```python
from build123d import *

# Parameters (mm, degrees)
SKETCH4_W            = 28.705590634
SKETCH4_H            = 208.526976526
BOSS_EXTRUDE5_DEPTH  = 20
SKETCH5_W            = 28.705590634
SKETCH5_H            = 20.449519005
SKETCH5_W_2          = 31.445291082
SKETCH5_H_2          = 18.706651284
BOSS_EXTRUDE6_DEPTH  = 40
SKETCH6_W            = 31.445291082
SKETCH6_H            = 208.079798694
BOSS_EXTRUDE7_DEPTH  = 40
SKETCH7_W            = 18.3
SKETCH7_H            = 20
CUT_EXTRUDE1_DEPTH   = 28.705590634
SKETCH8_W            = 208.079798694
SKETCH8_H            = 10.562870441
SKETCH8_H_2          = 11.993481809
BOSS_EXTRUDE8_DEPTH  = 15
SKETCH11_W           = 20
SKETCH11_H           = 32
CUT_EXTRUDE2_DEPTH   = 39
SKETCH12_W           = 21.023017078
SKETCH12_H           = 19.656473247
SKETCH12_W_2         = 18.706651284
SKETCH12_H_2         = 20
BOSS_EXTRUDE10_DEPTH = 68
SKETCH13_W           = 19.268882627
SKETCH13_H           = 20
SKETCH13_W_2         = 20.449519005
BOSS_EXTRUDE11_DEPTH = 64


with BuildPart() as part:
    # Sketch4 → Boss-Extrude5 (new body)
    with BuildSketch(Plane(origin=(0, -18, 0), x_dir=(1, 0, 0), z_dir=(0, 1, 0))):
        with Locations((-364.278541189, -59.921815566)):
            Rectangle(SKETCH4_W, SKETCH4_H)
    extrude(amount=BOSS_EXTRUDE5_DEPTH)

    # Sketch5 → Boss-Extrude6 (add)
    with BuildSketch(Plane.XZ.offset(18)):
        with Locations((-364.278541189, 153.960544327)):
            Rectangle(SKETCH5_W, SKETCH5_H)
        with Locations((-365.648391413, -34.988347055)):
            Rectangle(SKETCH5_W_2, SKETCH5_H_2)
    extrude(amount=BOSS_EXTRUDE6_DEPTH)

    # Sketch6 → Boss-Extrude7 (add)
    with BuildSketch(Plane.XZ.offset(58)):
        with Locations((-365.648391413, 60.145404482)):
            Rectangle(SKETCH6_W, SKETCH6_H)
    extrude(amount=BOSS_EXTRUDE7_DEPTH)

    # Sketch7 → Cut-Extrude1 (cut)
    with BuildSketch(Plane.ZY.offset(378.631336506)):
        with Locations((61.073274434, -8)):
            Rectangle(SKETCH7_W, SKETCH7_H)
    extrude(amount=-CUT_EXTRUDE1_DEPTH, mode=Mode.SUBTRACT)

    # Sketch8 → Boss-Extrude8 (add)
    with BuildSketch(Plane.ZY.offset(378.631336506)):
        with Locations((60.145404482, -63.281435221)):
            Rectangle(SKETCH8_W, SKETCH8_H)
        with Locations((60.145404482, -92.003259095)):
            Rectangle(SKETCH8_W, SKETCH8_H_2)
    extrude(amount=BOSS_EXTRUDE8_DEPTH)

    # Sketch11 → Cut-Extrude2 (cut)
    with BuildSketch(Plane.ZY.offset(393.631336506)):
        with Locations((145.629013926, -78.238745267)):
            Rectangle(SKETCH11_W, SKETCH11_H)
        with Locations((-23.889291997, -78.292410405)):
            Rectangle(SKETCH11_W, SKETCH11_H)
    extrude(amount=-CUT_EXTRUDE2_DEPTH, mode=Mode.SUBTRACT)

    # Sketch12 → Boss-Extrude10 (add)
    with BuildSketch(Plane.ZY.offset(378.631336506)):
        with Locations((153.67379529, -7.828236624)):
            Rectangle(SKETCH12_W, SKETCH12_H)
        with Locations((-34.988347055, -8)):
            Rectangle(SKETCH12_W_2, SKETCH12_H_2)
    extrude(amount=BOSS_EXTRUDE10_DEPTH)

    # Sketch13 → Boss-Extrude11 (add)
    with BuildSketch(Plane(origin=(-349.925745872, 0, 0), x_dir=(0, 0, -1), z_dir=(1, 0, 0))):
        with Locations((34.707231384, -8)):
            Rectangle(SKETCH13_W, SKETCH13_H)
        with Locations((-153.960544327, -8)):
            Rectangle(SKETCH13_W_2, SKETCH13_H)
    extrude(amount=BOSS_EXTRUDE11_DEPTH)


solid = part.part
```
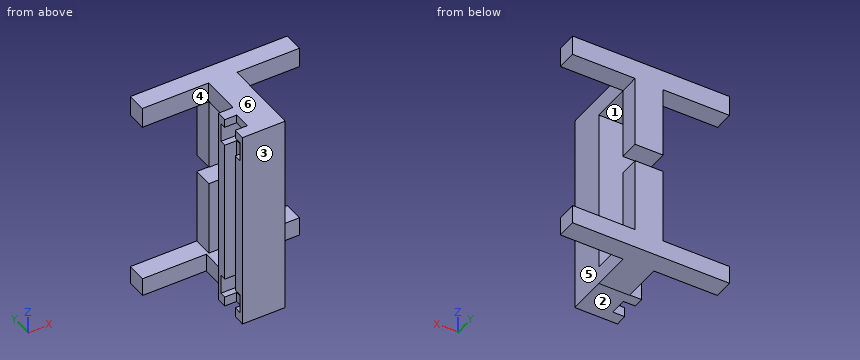
Design review of the part built by this model. Coordinates are the model's own, in mm. Face numbers are marked on the shaded views. A direction names the side the tool comes from. Round coordinates to 2 decimals unless told otherwise and drop trailing zeros. Write each loop counter-clockwise with the first axis right and the second up, starting at its lowest first coordinate (ties: lowest second). Pieces come first, ordered by that corner, then holes.
Item 1: We need section C-C on z = 22. Write out the cut boundary in (x, y).
Item 2: Clearance check with flat-ended pins moving along their axes: pin 1 Ø3 at (y, z) = (-83.5, 117.5) entering from -X; pin 2 Ø16 at (y, z) = (-3.5, 30.5) entering from +X; pin 3 Ø16 at (x, y) = (-370, -71.5) entering from -Z. State where each tip first meets the part, or that it passes through.
Item 3: We need section B-B on y = -24.5. Write out the cut boundary in (x, z), and give its area (3 significant figures).
Item 4: For the marked faces 4, 5 and 6, list the 3-axis set-ups (+Z, -Z, +X, -X, +Y, -Y) from which the entire face can be reached by the end or side of a thin tool; tool diameter is ignored.
Item 5: We need section A-A on x = -337. Write out the cut boundary in (y, z).
Item 6: The part is to be moulded in two halves that separate along Z. For the marked faces 1, 2 and 3, say which applies: +Z half, -Z half, draft (parallel to the pull), parting line (faces both ways), or undercut.
Item 7: We need section D-D on z = 148.5. Write out the cut boundary in (x, y).
Item 8: For probe 1 along Z at (x, y) = (-365.5, -89); probe 2 along Y at (x, z) = (-363.5, 121); probe 3 along Z at (x, y) = (-374, -5), list the stretches that pass through material, from the lowest coordinate up.
Returned:
1. outline: (-393.63, -98) - (-349.93, -98) - (-349.93, -58) - (-393.63, -58) - (-393.63, -68.56) - (-381.37, -68.56) - (-381.37, -86.01) - (-393.63, -86.01) - close; (-378.63, -18) - (-349.93, -18) - (-349.93, 2) - (-378.63, 2) - close
2. pin 1: stops at x = -381.37
2. pin 2: stops at x = -349.93
2. pin 3: stops at z = -43.89
3. outline: (-381.37, -44.34) - (-349.93, -44.34) - (-349.93, -25.64) - (-381.37, -25.64) - close; (-378.63, 143.74) - (-349.93, 143.74) - (-349.93, 164.19) - (-378.63, 164.19) - close
3. area: 1,180 mm2
4. face 4: +Z, -X
4. face 5: +Z, -Z, +X, -Y
4. face 6: +Z, +X, -X, +Y, -Y
5. outline: (-18, -44.34) - (2, -44.34) - (2, -25.07) - (-18, -25.07) - close; (-18, 143.74) - (2, 143.74) - (2, 164.19) - (-18, 164.19) - close
6. face 1: undercut
6. face 2: -Z half
6. face 3: draft
7. outline: (-446.63, -17.66) - (-378.63, -17.66) - (-378.63, -58) - (-393.63, -58) - (-393.63, -62.24) - (-354.63, -62.24) - (-354.63, -94.24) - (-393.63, -94.24) - (-393.63, -98) - (-349.93, -98) - (-349.93, -18) - (-285.93, -18) - (-285.93, 2) - (-446.63, 2) - close
8. probe 1: z = -43.89 to -33.89, -13.89 to 135.63, 155.63 to 164.19
8. probe 2: y = -98 to -58, -18 to 2
8. probe 3: z = -44.34 to 51.92, 70.22 to 164.19
